from build123d import *

# Parameters (mm, degrees)
SKETCH1_R           = 15.875
SKETCH1_R_2         = 2.38125
BOSS_EXTRUDE2_DEPTH = 3.175
SKETCH2_R           = 26.68586127
SKETCH2_R_2         = 15.875
CUT_EXTRUDE1_DEPTH  = 31.120694713


with BuildPart() as part:
    # Sketch1 → Boss-Extrude2 (new body)
    with BuildSketch(Plane.XY):
        with Locations((0, 9.525)):
            Circle(SKETCH1_R)
        Circle(SKETCH1_R_2, mode=Mode.SUBTRACT)
        with Locations((0, 19.05)):
            Circle(SKETCH1_R_2, mode=Mode.SUBTRACT)
    extrude(amount=BOSS_EXTRUDE2_DEPTH)

    # Sketch2 → Cut-Extrude1 (cut, through all)
    # profile 1 of 5: a face of its own
    with BuildSketch(Plane.XY.offset(3.175)):
        with Locations((0, 9.525)):
            Circle(SKETCH2_R)
        with Locations((0, 9.525)):
            Circle(SKETCH2_R_2, mode=Mode.SUBTRACT)
    # profile 2 of 5: a face of its own
    with BuildSketch(Plane.XY.offset(3.175)):
        with BuildLine():
            ThreePointArc((-4.130251428, 23.873227461), (-2.201704524, 25.006089085), (0, 25.4))
            ThreePointArc((0, 25.4), (-7.099515829, 23.724031657), (-12.7, 19.05))
            ThreePointArc((-12.7, 19.05), (-8.178609866, 21.041380315), (-4.130251428, 23.873227461))
        make_face()
    # profile 3 of 5: a face of its own
    with BuildSketch(Plane.XY.offset(3.175)):
        with BuildLine():
            ThreePointArc((4.130251428, 23.873227461), (8.178609866, 21.041380315), (12.7, 19.05))
            ThreePointArc((12.7, 19.05), (7.099515829, 23.724031657), (0, 25.4))
            ThreePointArc((0, 25.4), (2.201704524, 25.006089085), (4.130251428, 23.873227461))
        make_face()
    # profile 4 of 5: a face of its own
    with BuildSketch(Plane.XY.offset(3.175)):
        with BuildLine():
            ThreePointArc((-3e-09, -6.35), (7.099515827, -4.674031658), (12.7, 0))
            ThreePointArc((12.7, 0), (8.178609866, -1.991380315), (4.130251428, -4.823227461))
            ThreePointArc((4.130251428, -4.823227461), (2.201704523, -5.956089085), (-3e-09, -6.35))
        make_face()
    # profile 5 of 5: a face of its own
    with BuildSketch(Plane.XY.offset(3.175)):
        with BuildLine():
            ThreePointArc((-12.7, 0), (-7.09951583, -4.674031657), (-3e-09, -6.35))
            ThreePointArc((-3e-09, -6.35), (-2.201704525, -5.956089084), (-4.130251428, -4.823227461))
            ThreePointArc((-4.130251428, -4.823227461), (-8.178609866, -1.991380315), (-12.7, 0))
        make_face()
    extrude(amount=-CUT_EXTRUDE1_DEPTH, mode=Mode.SUBTRACT)


solid = part.part
Input: part model. Units: mm. Frame: model coordinates. Round coordinates to 2 decimals unless told otherwise and drop trailing zeros. Order: outer loops, then holes, each group sorted by start corner. A loop starts at its lowest first (then second) coordinate and runs counter-clockwise, first axis right, second up.
1. Material intervals for line 1 (Y direction, x = 0, z = 1.85); line 2 (Y direction, x = -2, z = 2.5); line 3 (X direction, y = -2, z = 2.25), sorted ascending.
The answers:
line 1: y = -6.35 to -2.38, 2.38 to 16.67, 21.43 to 25.4
line 2: y = -6.03 to -1.29, 1.29 to 17.76, 20.34 to 25.08
line 3: x = -8.16 to -1.29, 1.29 to 8.16
2. Cut plane A-A, the plane z = 0.6. State how many separate pieces and enclosed holes the cut face has, then the cut area to 3 significant figures.
The answers:
separate pieces: 1
enclosed holes: 2
area: 698 mm2
3. Pin query (flat end, axial travel): P1, Ø1, axis at x = 4, z = 0.5, coming from the -Y side; P2, Ø1, axis at y = 15, z = 0.5, coming from the +X side; P3, Ø4, axis at x = 0, y = 0, coming from the -Z side. Return the tip coordinate at first contact, or that it passes through.
The answers:
P1: stops at y = -5.3
P2: stops at x = 15.08
P3: passes through
4. Cut plane D-D, the plane x = -5.5. Output: boundary loops of the cut face in (y, z) (3 decimals), then the cut area to 3 significant figures.
The answers:
outline: (-3.73, 0) - (22.78, 0) - (22.78, 3.175) - (-3.73, 3.175) - close
area: 84.2 mm2
5. Cut plane B-B, the plane y = -1.5. Output: boundary loops of the cut face in (x, z) (3 decimals), then the cut area to 3 significant figures.
The answers:
outline: (-9.095, 0) - (-1.849, 0) - (-1.849, 3.175) - (-9.095, 3.175) - close; (1.849, 0) - (9.095, 0) - (9.095, 3.175) - (1.849, 3.175) - close
area: 46.0 mm2
6. Cut plane C-C, the plane x = 0.5. Output: boundary loops of the cut face in (y, z) (3 decimals), then the cut area to 3 significant figures.
The answers:
outline: (-6.33, 0) - (-2.328, 0) - (-2.328, 3.175) - (-6.33, 3.175) - close; (2.328, 0) - (16.722, 0) - (16.722, 3.175) - (2.328, 3.175) - close; (21.378, 0) - (25.38, 0) - (25.38, 3.175) - (21.378, 3.175) - close
area: 71.1 mm2
